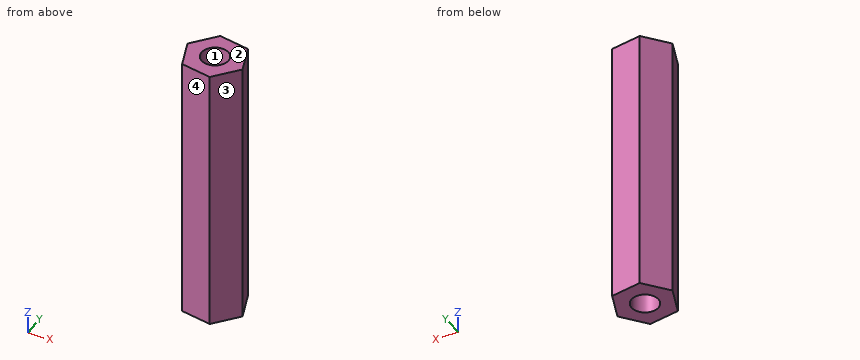
from build123d import *

# Parameters (mm, degrees)
RESSALTO_EXTRUS_O1_DEPTH = 30
ESBO_O4_R                = 1.5
CORTE_EXTRUS_O2_DEPTH    = 40


with BuildPart() as part:
    # Esboço1 → Ressalto-extrusão1 (new body)
    with BuildSketch(Plane.XY):
        Polygon((12.933175524, -4.143885809), (9.525050306, -3.523658029), (7.283854683, -6.165067156), (8.450784277, -9.426704064), (11.858909495, -10.046931845), (14.100105118, -7.405522718), align=None)
    extrude(amount=RESSALTO_EXTRUS_O1_DEPTH)

    # Esboço4 → Corte-extrusão2 (cut)
    with BuildSketch(Plane(origin=(0, 0, 0), x_dir=(-1, 0, 0), z_dir=(0, 0, -1))):
        with Locations((-10.691979901, -6.785294937)):
            Circle(ESBO_O4_R)
    extrude(amount=-CORTE_EXTRUS_O2_DEPTH, mode=Mode.SUBTRACT)


solid = part.part
Geometry check sheet. Reference: the model listing, model coordinates, mm. Face numbers are marked on the shaded views. Give positions to 0.01 mm unless a question says otherwise; leave off trailing zeros. Write each loop counter-clockwise with the first axis right and the second up, starting at its lowest first coordinate (ties: lowest second). Pieces come first, ordered by that corner, then holes. Notation, with made-up numbers: (5.5, 48.5) - (29.5, 48.5) arc R28 ccw to (29.5, 69.5) - close; hole circle Ø2 at (54.25, 50). An arc over 180 degrees is marked (long way). Put each result on its own line as item: value.
1. Sectioned sample at B-B, the plane x = 10.5. Enter the section's corners in (y, z).
Ans:
outline: (-9.8, 0) - (-8.27, 0) - (-8.27, 30) - (-9.8, 30) - close; (-5.3, 0) - (-3.7, 0) - (-3.7, 30) - (-5.3, 30) - close
2. Go/stop test with flat-tipped pins: pin 1 (2 mm diameter, centred on y = -8, z = 10.5, fed in from -X); pin 2 (2.5 mm diameter, centred on x = 10.69, y = -6.79, fed in from +Z); pin 3 (1.5 mm diameter, centred on x = 13, z = 5.5, fed in from -Y); pin 4 (4 mm diameter, centred on x = 9.5, z = 21, fed in from +Y). Record where each tip stops, or that it passes through.
Ans:
pin 1: stops at x = 7.58
pin 2: passes through
pin 3: stops at y = -9.59
pin 4: stops at y = -3.52
3. Thickness scan on line 1 (Y direction, x = 10, z = 15.25); line 2 (X direction, y = -6.5, z = 24.5); line 3 (Y direction, x = 11.75, z = 7.25). Record the ranges inside material, lowest first.
Ans:
line 1: y = -9.71 to -8.12, -5.45 to -3.61
line 2: x = 7.4 to 9.22, 12.16 to 13.78
line 3: y = -10.03 to -7.85, -5.72 to -3.93
4. Sectioned sample at C-C, the plane z = 6.5. Enter the section's corners in (x, y).
Ans:
outline: (7.28, -6.17) - (8.45, -9.43) - (11.86, -10.05) - (14.1, -7.41) - (12.93, -4.14) - (9.53, -3.52) - close; hole circle Ø3 at (10.69, -6.79)
5. Sectioned sample at A-A, the plane y = -5.75. Enter the section's corners in (x, z), plus the area to 3 significant figures.
Ans:
outline: (7.64, 0) - (9.61, 0) - (9.61, 30) - (7.64, 30) - close; (11.78, 0) - (13.51, 0) - (13.51, 30) - (11.78, 30) - close
area: 111 mm²
6. Draft check along X on the marked faces 1, 2, 3 and 4. Enter one of: +X half, -X half, draft (parallel to the pull), parting line (faces both ways), or undercut.
Ans:
face 1: undercut
face 2: draft
face 3: +X half
face 4: -X half
